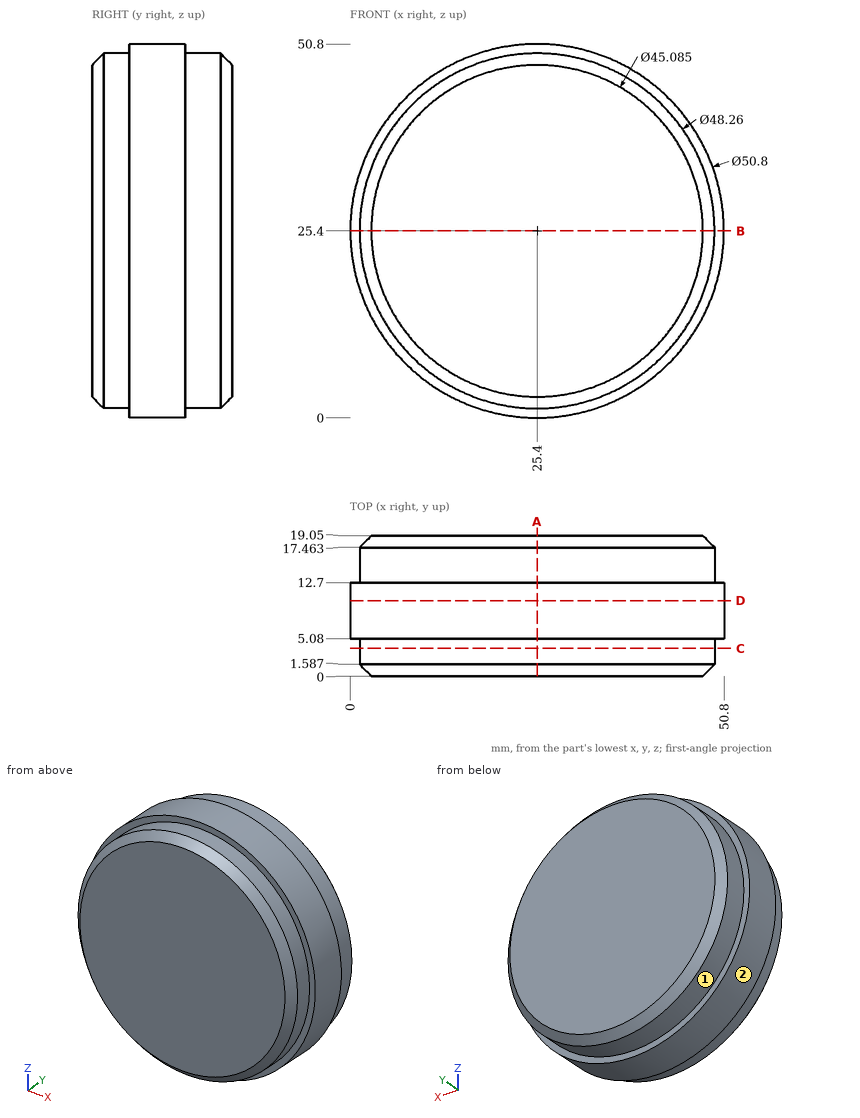
Answer from the drawing. Dimensions are ordinates in mm from the lowest x, y and z of the part. A direction names the side the tool comes from. Give positions to 0.01 mm unless a question says otherwise; leave off trailing zeros. Order: outer loops, then holes, each group sorted by start corner. A loop starts at its lowest first (then second) coordinate and runs counter-clockwise, first axis right, second up. Notation, with made-up numbers: (21, -35.75) -> (36, -35.75) arc R20 cw to (36, -2.75) -> close; hole circle Ø9 at (42, 2.25). An arc over 180 degrees is marked (long way). Answer as a JSON object with one key per item and string values. Group by question number.
1. Section A-A on x = 25.4 is taken. Determine the outline of the cut face in (y, z).
2. A tool of negligible diameter and unlimited length cuts with its end or side. For the marked faces 1 and 2, from which of +Z, -Z, +X, -X, +Y, -Y can it reach the whole face along a straight path? Write none if from no direction.
3. Section B-B on z = 25.4 is taken. Determine the outline of the cut face in (x, y).
4. A flat-ended cylindrical pin translates along its axis: pin 1 Ø5 at (x, y) = (10, 9.5) entering from -Z. Find the tip coordinate at first contact, or state that the pin passes through.
5. Consider line 1 along X through (y, z) = (10.25, 17.5); line 2 along X through (y, z) = (11.5, 25.5); line 3 along Z through (x, y) = (44.5, 11.5) (1 decimal). Determine where each line is inside the solid, lowest interval first. Write a range as [from, to].
6. Section D-D on y = 10.25 is taken. Determine the outline of the cut face in (x, z), plus the area to 3 significant figures.
7. Section C-C on y = 3.75 is taken. Determine the outline of the cut face in (x, z).
Result sheet:
{
 "1": {"outline": "(0, 2.86) -> (1.59, 1.27) -> (5.08, 1.27) -> (5.08, 0) -> (12.7, 0) -> (12.7, 1.27) -> (17.46, 1.27) -> (19.05, 2.86) -> (19.05, 47.94) -> (17.46, 49.53) -> (12.7, 49.53) -> (12.7, 50.8) -> (5.08, 50.8) -> (5.08, 49.53) -> (1.59, 49.53) -> (0, 47.94) -> close"},
 "2": {"face 1": "+Y", "face 2": "+Y, -Y"},
 "3": {"outline": "(0, 5.08) -> (1.27, 5.08) -> (1.27, 1.59) -> (2.86, 0) -> (47.94, 0) -> (49.53, 1.59) -> (49.53, 5.08) -> (50.8, 5.08) -> (50.8, 12.7) -> (49.53, 12.7) -> (49.53, 17.46) -> (47.94, 19.05) -> (2.86, 19.05) -> (1.27, 17.46) -> (1.27, 12.7) -> (0, 12.7) -> close"},
 "4": {"pin 1": "stops at z = 3.52"},
 "5": {"line 1": "x = [1.26, 49.54]", "line 2": "x = [0, 50.8]", "line 3": "z = [8.7, 42.1]"},
 "6": {"outline": "circle Ø50.8 at (25.4, 25.4)", "area": "2,030 mm^2"},
 "7": {"outline": "circle Ø48.26 at (25.4, 25.4)"}
}
